```python
from build123d import *

# Parameters (mm, degrees)
F1_DEPTH = 6.35
F2_T     = 0.762


with BuildPart() as f1:
    # F0 (on Top) → F1 (new body)
    with BuildSketch(Plane.XY):
        with BuildLine():
            Line((-44.2468, -31.75), (0, -31.75))
            ThreePointArc((0, -31.75), (31.75, 0), (0, 31.75))
            Line((0, 31.75), (-44.2468, 31.75))
            ThreePointArc((-44.2468, 31.75), (-75.9968, 0), (-44.2468, -31.75))
        make_face()
    extrude(amount=F1_DEPTH)

    # F2
    f2_openings = [f1.faces().sort_by_distance(p)[0] for p in [
        (-22.1234, 0, 6.35),
    ]]
    offset(amount=F2_T, openings=f2_openings, kind=Kind.INTERSECTION)


solid = f1.part
```
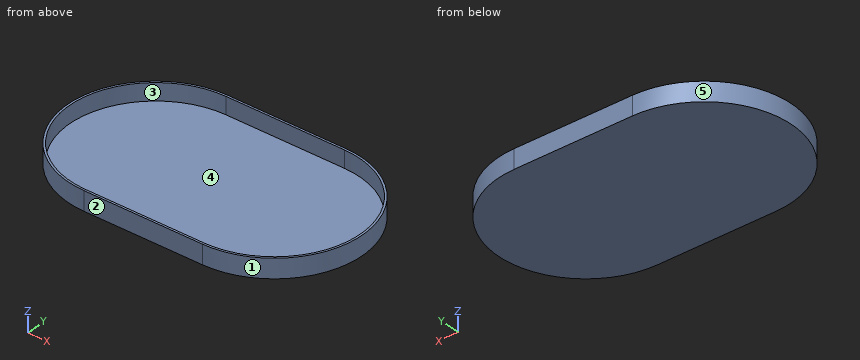
Can you work these out from the model? Positions are in its coordinate system, mm. Face numbers are marked on the shaded views. A direction names the side the tool comes from. Give positions to 0.01 mm unless a question says otherwise; leave off trailing zeros. Order: outer loops, then holes, each group sorted by start corner. A loop starts at its lowest first (then second) coordinate and runs counter-clockwise, first axis right, second up. Notation, with made-up numbers: M 22,29.5 L 60,29.5 A13 ccw 60,33.5 Z; hole C 84.5,38.25 d9. An arc over 180 degrees is marked long. One line per item, written item: value.
1) On a 3-axis mill with a long thin cutter (end or side, diameter ignored), from which of +Z, -Z, +X, -X, +Y, -Y can I reach the whole of each face in a straight line? I mean the marked faces 4 and 5. Say none if no direction works.
Answer sheet:
face 4: +Z
face 5: +Z, -Z, -X
2) I want a section at A-A, the plane z = 3.25. List the corners of the cut face in (x, y) for me.
Answer sheet:
outline: M -44.25,-32.51 L 0,-32.51 A32.51 ccw 0,32.51 L -44.25,32.51 A32.51 ccw Z; hole M -44.25,-31.75 L 0,-31.75 A31.75 ccw 0,31.75 L -44.25,31.75 A31.75 ccw Z
3) I want a section at B-B, the plane y = 0. List the corners of the cut face in (x, z) for me.
Answer sheet:
outline: M -76.76,-0.76 L 32.51,-0.76 L 32.51,6.35 L 31.75,6.35 L 31.75,0 L -76,0 L -76,6.35 L -76.76,6.35 Z
4) We'd pull the mould along Y, two halves only. Please class the marked faces 1, 2 and 3: released by +Y, released by -Y, zero draft, split by the parting line, or undercut.
Answer sheet:
face 1: split by the parting line
face 2: released by -Y
face 3: undercut
5) I want a section at C-C, the plane x = -6. List the corners of the cut face in (y, z) for me, plus the area to 3 significant figures.
Answer sheet:
outline: M -32.51,-0.76 L 32.51,-0.76 L 32.51,6.35 L 31.75,6.35 L 31.75,0 L -31.75,0 L -31.75,6.35 L -32.51,6.35 Z
area: 59.2 mm^2
6) Please list where these lines run through material, in increasing order: line 1 along Y through (x, z) = (-24, 3); line 2 along Z through (x, y) = (-55.5, -22.5); line 3 along Y through (x, z) = (25, 0.25).
Answer sheet:
line 1: y = -32.51 to -31.75, 31.75 to 32.51
line 2: z = -0.76 to 0
line 3: y = -20.79 to -19.57, 19.57 to 20.79
7) For P1, Ø1, axis at x = -4.5, y = -14, coming from the +Z side; P2, Ø2, axis at y = -10.5, z = 1, coming from the -X side; P3, Ø4, axis at y = -3.5, z = 1.5, coming from the -X side, each with a flat end and sliding along its axis, tell me the tip position at first contact or that it passes through.
Answer sheet:
P1: stops at z = 0
P2: stops at x = -75.34
P3: stops at x = -76.72
